Part model, mm, in its own coordinate system. A direction names the side the tool comes from. Round coordinates to 2 decimals unless told otherwise and drop trailing zeros. Loops run counter-clockwise (first coordinate to the right, second up) from the corner with the lowest first, then second, coordinate; pieces in that order, holes last.
1) Mould opens along Y. For faces 3 (the cylindrical face through (0, 2, 4)), 4 (the cylindrical face through (3.684, -123.408, 3.451)), 5 (the flat face through (2, -57, 7)) say: +Y half, -Y half, draft (parallel to the pull), parting line (faces both ways), or undercut.
2) Probe line 1 (Y direction, x = 3.25, z = 0.75); line 2 (X direction, y = -38, z = 4.25); line 3 (X direction, y = -45.5, z = 6.5). List the from-to ranges inside material, lowest first.
3) 3-axis set-ups, long thin cutter, end or side, ignore diameter. For faces 1 (the flat face through (-2.5, -19, 3)), 2 (the cylindrical face through (3.5, -117.3, 3.5)): which of +Z, -Z, +X, -X, +Y, -Y reach the whole face in a straight line?
4) Band-saw the part on A-A, the plane x = 3.5. Write the cut outline in (y, z).
5) Band-saw the part on C-C, the plane y = -12.5. Write the cut outline in (x, z), then the cut area to 3 significant figures.
6) Band-saw the part on B-B, the plane z = 1.5. Write the cut outline in (x, y), then the cut area to 3 significant figures.
7) Band-saw the part on D-D, the plane x = -5.75. Write the cut outline in (y, z), then the cut area to 3 significant figures.
8) Drop flat-ended pins along their axis: P1, Ø2, axis at y = -19, z = 4, coming from the -X side; P2, Ø3.5, axis at x = 0, y = 0, coming from the -Z side; P3, Ø1, axis at x = -5, z = 1.5, coming from the +Y side. Give the stop position or say it passes through.
from build123d import *

# Parameters (mm, degrees)
F0_R     = 2
F1_DEPTH = 7
F2_D     = 4
F3_D     = 4


with BuildPart() as f1:
    # F0 (on Top) → F1 (new body)
    with BuildSketch(Plane.XY):
        with BuildLine():
            Line((7.5, -41), (7.5, 0))
            ThreePointArc((7.5, 0), (-4.3301270189, 6.123724357), (-2.5, -7.0710678119))
            Line((-2.5, -7.0710678119), (-2.5, -32.0124984811))
            ThreePointArc((-2.5, -32.0124984811), (-6.5397745633, -35.4838365332), (-7.2178157357, -40.7668495526))
            Line((-7.2178157357, -40.7668495526), (0, -121))
            ThreePointArc((0, -121), (3.75, -123.4084825035), (7.5, -121))
            Line((7.5, -121), (7.5, -41))
        make_face()
        with Locations((3.75, -119.2848719021)):
            Circle(F0_R, mode=Mode.SUBTRACT)
    extrude(amount=F1_DEPTH)

    # F2 (through all)
    with Locations(Plane(origin=(0, 0, 0), x_dir=(1, 0, 0), z_dir=(0, 0, -1))):
        with Locations((0, 0)):
            Hole(F2_D / 2)

    # F3 (through all)
    with Locations(Plane(origin=(0, 0, 0), x_dir=(1, 0, 0), z_dir=(0, 0, -1))):
        with Locations((0, 39.008192718)):
            Hole(F3_D / 2)


solid = f1.part
Reported:
1. face 3: undercut
1. face 4: -Y half
1. face 5: draft
2. line 1: y = -123.38 to -121.22, -117.35 to 6.76
2. line 2: x = -7.36 to -1.73, 1.73 to 7.5
2. line 3: x = -6.79 to 7.5
3. face 1: +Z, -Z, -X
3. face 2: +Z, -Z
4. outline: (-123.4, 0) - (-121.27, 0) - (-121.27, 7) - (-123.4, 7) - close; (-117.3, 0) - (6.63, 0) - (6.63, 7) - (-117.3, 7) - close
5. outline: (-2.5, 0) - (7.5, 0) - (7.5, 7) - (-2.5, 7) - close
5. area: 70.0 mm2
6. outline: (-7.22, -40.77) - (0, -121) arc R4.12 ccw to (7.5, -121) - (7.5, 0) arc R7.5 ccw (long way) to (-2.5, -7.07) - (-2.5, -32.01) arc R7.43 ccw to start; hole circle Ø4 at (0, -39.01); hole circle Ø4 at (0, 0); hole circle Ø4 at (3.75, -119.28)
6. area: 1,420 mm2
7. outline: (-57.08, 0) - (-34.3, 0) - (-34.3, 7) - (-57.08, 7) - close; (-4.82, 0) - (4.82, 0) - (4.82, 7) - (-4.82, 7) - close
7. area: 227 mm2
8. P1: stops at x = -2.5
8. P2: passes through
8. P3: stops at y = 6
